Check sheet for the drawn part. Datum: minimum x, y, z corner. Units: mm. Coordinates: 2 decimals unless noted, no trailing zeros. Loops run counter-clockwise (first coordinate to the right, second up) from the corner with the lowest first, then second, coordinate; pieces in that order, holes last.
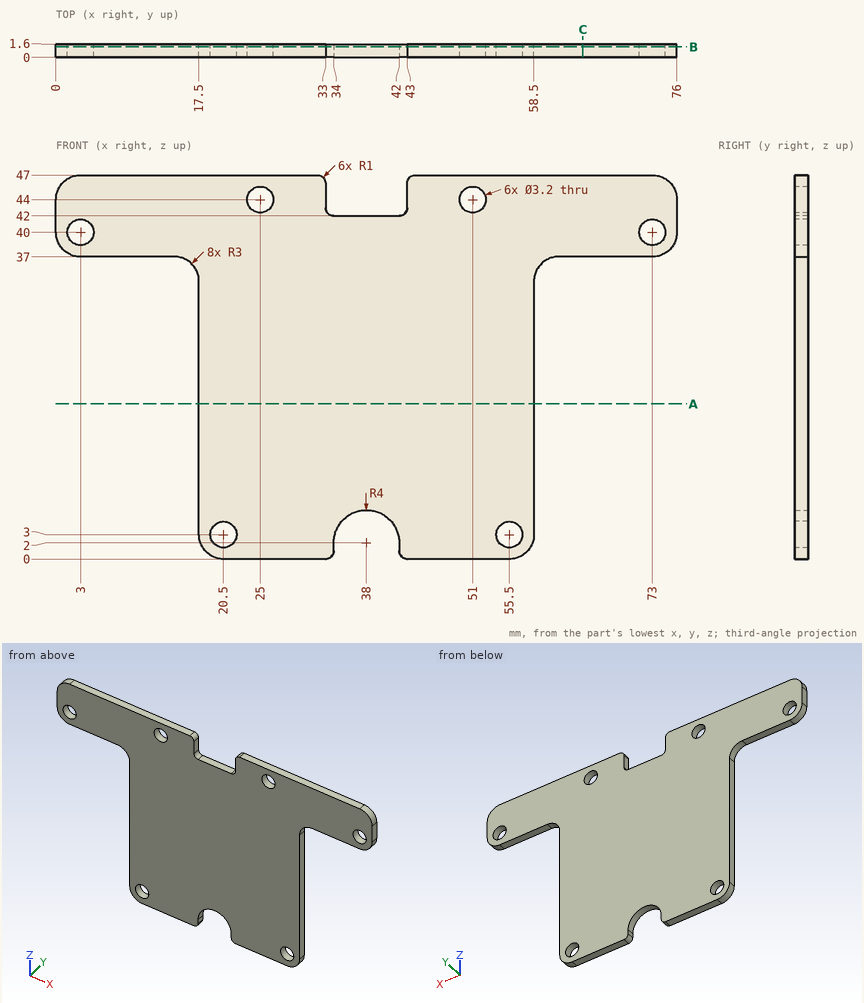
(1) Sectioned sample at C-C on x = 64.5. Record the cut outline in (y, z), and give its area (3 significant figures).
Findings:
outline: (0, 37) - (1.6, 37) - (1.6, 47) - (0, 47) - close
area: 16.0 mm2
(2) Gauge pin test, flat ends, axial feed: pin 1 Ø0.5 at (y, z) = (0.5, 1.5) entering from -X; pin 2 Ø0.8 at (y, z) = (0.5, 21.5) entering from -X; pin 3 Ø0.5 at (x, y) = (39.5, 1) entering from +Z. Record the tip position at first contact, or that the pin passes through.
Findings:
pin 1: stops at x = 17.77
pin 2: stops at x = 17.5
pin 3: stops at z = 42
(3) Scan lines: L1, parallel to X at y = 0.65, z = 40; L2, parallel to X at y = 1.1, z = 44; L3, parallel to X at y = 0.65, z = 28. Record each from-to range of solid material in increasing order.
Findings:
L1: x = 0 to 1.4, 4.6 to 71.4, 74.6 to 76
L2: x = 0 to 23.4, 26.6 to 33, 43 to 49.4, 52.6 to 76
L3: x = 17.5 to 58.5
(4) Sectioned sample at B-B on y = 1.25. State how many separate pieces and enclosed holes the cut face has, and give its area (3 significant figures).
Findings:
separate pieces: 1
enclosed holes: 6
area: 2,130 mm2
(5) Sectioned sample at A-A on z = 19. Record the cut outline in (x, y).
Findings:
outline: (17.5, 0) - (58.5, 0) - (58.5, 1.6) - (17.5, 1.6) - close
